Can you work these out from the model? Positions are in its coordinate system, mm. Face numbers are marked on the shaded views. A direction names the side the tool comes from. Round coordinates to 2 decimals unless told otherwise and drop trailing zeros. Loops run counter-clockwise (first coordinate to the right, second up) from the corner with the lowest first, then second, coordinate; pieces in that order, holes last. Notation, with made-up numbers: (-9.5, 64) - (21.5, 64) arc R23 cw to (21.5, 90) - close; hole circle Ø10 at (56, -2). An arc over 180 degrees is marked (long way). Answer as CSV lines item,"result".
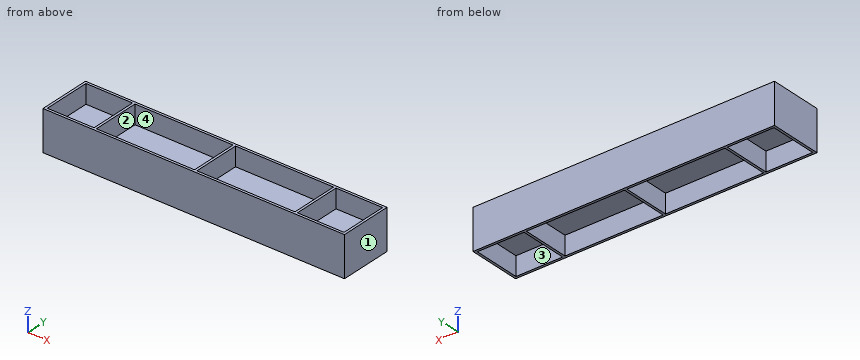
```python
from build123d import *

# Parameters (mm, degrees)
SKETCH_1_W           = 1500
SKETCH_1_H           = 262
EXTRUDE_1_DEPTH      = 200
SKETCH_5_W           = 232
SKETCH_5_H           = 238
SKETCH_5_W_2         = 488
CUT_EXTRUDE_10_DEPTH = 1536.787745751
SKETCH_7_W           = 1500
SKETCH_7_H           = 12
EXTRUDE_13_DEPTH     = 260


with BuildPart() as part:
    # 草图1 → 拉伸1 (new body)
    with BuildSketch(Plane.XY):
        with Locations((750, 131)):
            Rectangle(SKETCH_1_W, SKETCH_1_H)
    extrude(amount=EXTRUDE_1_DEPTH)

    # 草图5 → 拉伸10 (cut, through all)
    with BuildSketch(Plane.XY.offset(200)):
        with Locations((128, 131)):
            Rectangle(SKETCH_5_W, SKETCH_5_H)
        with Locations((500, 131)):
            Rectangle(SKETCH_5_W_2, SKETCH_5_H)
        with Locations((1000, 131)):
            Rectangle(SKETCH_5_W_2, SKETCH_5_H)
        with Locations((1372, 131)):
            Rectangle(SKETCH_5_W, SKETCH_5_H)
    extrude(amount=-CUT_EXTRUDE_10_DEPTH, mode=Mode.SUBTRACT)

    # 草图7 → 拉伸13 (add)
    with BuildSketch(Plane.XZ):
        with Locations((750, 100)):
            Rectangle(SKETCH_7_W, SKETCH_7_H)
    extrude(amount=-EXTRUDE_13_DEPTH)


solid = part.part
```
Q1. Imagine slicing it at B-B (x = 1335). Write out the boundary of the cut face in (y, z), then the cut area to 3 significant figures.
Checks:
outline,"(0, 0) - (12, 0) - (12, 94) - (250, 94) - (250, 0) - (262, 0) - (262, 200) - (250, 200) - (250, 106) - (12, 106) - (12, 200) - (0, 200) - close"
area,"7,660 mm²"
Q2. Imagine slicing it at A-A (z = 68.5). Write out the boundary of the cut face in (x, y).
Checks:
outline,"(0, 0) - (1500, 0) - (1500, 262) - (0, 262) - close; hole (12, 12) - (244, 12) - (244, 250) - (12, 250) - close; hole (256, 12) - (744, 12) - (744, 250) - (256, 250) - close; hole (756, 12) - (1244, 12) - (1244, 250) - (756, 250) - close; hole (1256, 12) - (1488, 12) - (1488, 250) - (1256, 250) - close"
Q3. If I drill on line 1 along X through (y, z) = (173, 148.5); line 2 along Y through (x, z) = (669.5, 27.5); line 3 along Z through (x, y) = (1258, 185.5), over which ranges is the centre line in solid material (lowest first)? Write a range as [from, to].
Checks:
line 1,"[0, 12], [244, 256], [744, 756], [1244, 1256], [1488, 1500]"
line 2,"[0, 12], [250, 262]"
line 3,"[94, 106]"
Q4. I'm going to push flat-ended pins straight in: pin 1 Ø8 at (x, y) = (564.5, 99.5) entering from -Z; pin 2 Ø6 at (x, y) = (1318.5, 75.5) entering from +Z. Where does each tip first touch, or does it pass through?
Checks:
pin 1,"z = 94"
pin 2,"z = 106"
Q5. We'd pull the mould along Y, two halves only. Please class the marked faces 1 and 2: pulls with the +Y half, pulls with the -Y half, needs draft (parallel to the pull), parting line crosses it, or undercut.
Checks:
face 1,"needs draft"
face 2,"undercut"
Q6. On a 3-axis mill with a long thin cutter (end or side, diameter ignored), from which of +Z, -Z, +X, -X, +Y, -Y can I reach the whole of each face in a straight line? I mean the marked faces 3 and 4. Say none if no direction works.
Checks:
face 3,"-Z"
face 4,"+Z"
